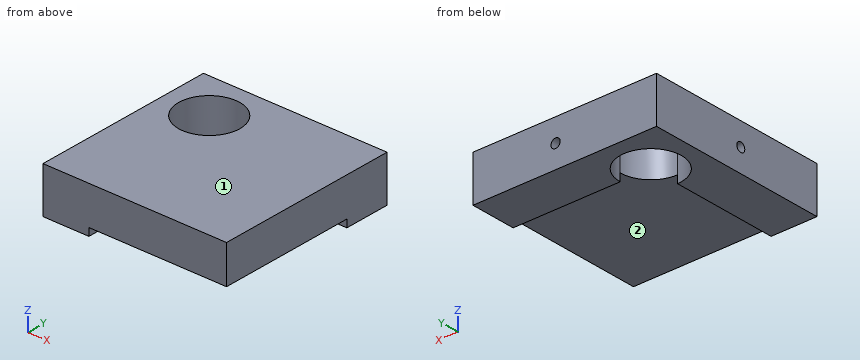
from build123d import *

# Parameters (mm, degrees)
F1_DEPTH = 19.05
F2_DEPTH = 3.175
F4_D     = 3.81
F4_DEPTH = 21.59
F4_TIP   = 1.1446394792
F6_D     = 3.81
F6_DEPTH = 21.59
F6_TIP   = 1.1446394792


with BuildPart() as f1:
    # F0 (on Top) → F1 (new body)
    with BuildSketch(Plane.XY):
        with BuildLine():
            Line((38.1, -42.2910004854), (38.1, 14.8589995146))
            Line((38.1, 14.8589995146), (-6.3500002354, 14.8589995146))
            ThreePointArc((-6.3500002354, 14.8589995146), (-10.0697441144, 5.8787433935), (-19.0500002354, 2.1589995146))
            Line((-19.0500002354, 2.1589995146), (-19.0500002354, -42.2910004854))
            Line((-19.0500002354, -42.2910004854), (38.1, -42.2910004854))
        make_face()
        with BuildLine():
            Line((38.1, 14.8589995146), (38.1, 33.9089995146))
            Line((38.1, 33.9089995146), (-38.1, 33.9089995146))
            Line((-38.1, 33.9089995146), (-38.1, -42.2910004854))
            Line((-38.1, -42.2910004854), (-19.0500002354, -42.2910004854))
            Line((-19.0500002354, -42.2910004854), (-19.0500002354, 2.1589995146))
            ThreePointArc((-19.0500002354, 2.1589995146), (-28.0302563565, 23.8392556356), (-6.3500002354, 14.8589995146))
            Line((-6.3500002354, 14.8589995146), (38.1, 14.8589995146))
        make_face()
    extrude(amount=F1_DEPTH)

    # F0 (on Top) → F2 (cut)
    with BuildSketch(Plane.XY):
        with BuildLine():
            Line((38.1, -42.2910004854), (38.1, 14.8589995146))
            Line((38.1, 14.8589995146), (-6.3500002354, 14.8589995146))
            ThreePointArc((-6.3500002354, 14.8589995146), (-10.0697441144, 5.8787433935), (-19.0500002354, 2.1589995146))
            Line((-19.0500002354, 2.1589995146), (-19.0500002354, -42.2910004854))
            Line((-19.0500002354, -42.2910004854), (38.1, -42.2910004854))
        make_face()
    extrude(amount=F2_DEPTH, mode=Mode.SUBTRACT)

    # F4
    with Locations(Plane(origin=(-38.1, 0, 0), x_dir=(0, -1, 0), z_dir=(-1, 0, 0))):
        with Locations((6.0960004854, 9.525)):
            Hole(F4_D / 2, depth=F4_DEPTH)
            with Locations((0, 0, -(F4_DEPTH + F4_TIP / 2))):  # 118° drill point
                Cone(0, F4_D / 2, F4_TIP, mode=Mode.SUBTRACT)

    # F6
    with Locations(Plane(origin=(0, 33.9089995146, 0), x_dir=(-1, 0, 0), z_dir=(0, 1, 0))):
        with Locations((-3.81, 9.525)):
            Hole(F6_D / 2, depth=F6_DEPTH)
            with Locations((0, 0, -(F6_DEPTH + F6_TIP / 2))):  # 118° drill point
                Cone(0, F6_D / 2, F6_TIP, mode=Mode.SUBTRACT)


solid = f1.part
Input: part model. Units: mm. Frame: model coordinates. Face numbers are marked on the shaded views. A direction names the side the tool comes from. Round coordinates to 2 decimals unless told otherwise and drop trailing zeros. Order: outer loops, then holes, each group sorted by start corner. A loop starts at its lowest first (then second) coordinate and runs counter-clockwise, first axis right, second up.
1. Cut plane C-C, the plane x = 13. Output: boundary loops of the cut face in (y, z) (3 decimals), then the cut area to 3 significant figures.
The answers:
outline: (-42.291, 3.175) - (14.859, 3.175) - (14.859, 0) - (33.909, 0) - (33.909, 19.05) - (-42.291, 19.05) - close
area: 1,270 mm2
2. Cut plane A-A, the plane y = -14. Output: boundary loops of the cut face in (x, z) (3 decimals).
The answers:
outline: (-38.1, 0) - (-19.05, 0) - (-19.05, 3.175) - (38.1, 3.175) - (38.1, 19.05) - (-38.1, 19.05) - close
3. Pin query (flat end, axial travel): P1, Ø2.5, axis at x = 15, z = 1.5, coming from the -Y side; P2, Ø1, axis at x = -9.5, y = 9, coming from the -Z side. Return the tip coordinate at first contact, or that it passes through.
The answers:
P1: stops at y = 14.86
P2: passes through
4. Set-up query: the marked faces 1 and 2. Return all of +Z, -Z, +X, -X, +Y, -Y with unobstructed straight access to the full face (end or side cutting, diameter ignored); none if empty.
The answers:
face 1: +Z, +X, -X, +Y, -Y
face 2: -Z, +X, -Y
5. Cut plane B-B, the plane z = 14.75. Output: boundary loops of the cut face in (x, y), then the cut area to 3 significant figures.
The answers:
outline: (-38.1, -42.29) - (38.1, -42.29) - (38.1, 33.91) - (-38.1, 33.91) - close; hole circle Ø25.4 at (-19.05, 14.86)
area: 5,300 mm2
6. Cut plane D-D, the plane z = 2.25. Output: boundary loops of the cut face in (x, y).
The answers:
outline: (-38.1, -42.29) - (-19.05, -42.29) - (-19.05, 2.16) arc R12.7 cw (long way) to (-6.35, 14.86) - (38.1, 14.86) - (38.1, 33.91) - (-38.1, 33.91) - close
7. Material intervals for line 1 (Z direction, x = 31.5, y = -21.5) (3 decimals); line 2 (X direction, y = 26, z = 10); line 3 (Y direction, x = -19.05, z = 14), sorted ascending.
The answers:
line 1: z = 3.175 to 19.05
line 2: x = -38.1 to -25.15, -12.95 to 1.97, 5.65 to 38.1
line 3: y = -42.29 to 2.16, 27.56 to 33.91
